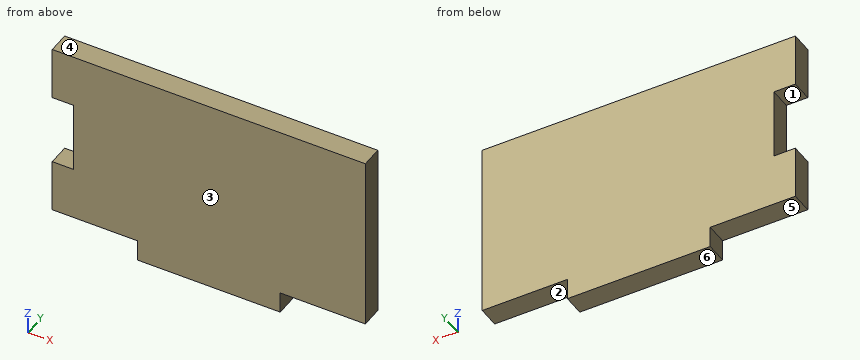
from build123d import *

# Parameters (mm, degrees)
SKETCH1_W           = 23.83759514
SKETCH1_H           = 6
SKETCH1_W_2         = 40
SKETCH1_W_3         = 23.837595139
BOSS_EXTRUDE1_DEPTH = 50
SKETCH1_3_W         = 40
SKETCH1_3_H         = 6
BOSS_EXTRUDE2_DEPTH = 6
SKETCH2_W           = 6
SKETCH2_H           = 20
CUT_EXTRUDE1_DEPTH  = 6


with BuildPart() as part:
    # Sketch1 → Boss-Extrude1 (new body)
    with BuildSketch(Plane.XY):
        with Locations((-42.937060586, -38.008278224)):
            Rectangle(SKETCH1_W, SKETCH1_H)
        with Locations((-11.018263016, -38.008278224)):
            Rectangle(SKETCH1_W_2, SKETCH1_H)
        with Locations((20.900534554, -38.008278224)):
            Rectangle(SKETCH1_W_3, SKETCH1_H)
    extrude(amount=BOSS_EXTRUDE1_DEPTH)

    # Sketch1_3 → Boss-Extrude2 (add)
    with BuildSketch(Plane.XY):
        with Locations((-11.018263016, -38.008278224)):
            Rectangle(SKETCH1_3_W, SKETCH1_3_H)
    extrude(amount=-BOSS_EXTRUDE2_DEPTH)

    # Sketch2 → Cut-Extrude1 (cut)
    with BuildSketch(Plane(origin=(0, -35.008278224, 0), x_dir=(1, 0, 0), z_dir=(0, 1, 0))):
        with Locations((-51.855858156, -25)):
            Rectangle(SKETCH2_W, SKETCH2_H)
    extrude(amount=-CUT_EXTRUDE1_DEPTH, mode=Mode.SUBTRACT)


solid = part.part
Can you work these out from the model? Positions are in its coordinate system, mm. Face numbers are marked on the shaded views. A direction names the side the tool comes from. Round coordinates to 2 decimals unless told otherwise and drop trailing zeros. Order: outer loops, then holes, each group sorted by start corner. A loop starts at its lowest first (then second) coordinate and runs counter-clockwise, first axis right, second up. Notation, with made-up numbers: (35, -37) -> (77, -37) arc R11 cw to (77, -19) -> close; hole circle Ø8 at (66.25, -7.75). An arc over 180 degrees is marked (long way). Write each question's results on one line, items separated by ' | '. Start each with the question number.
Item 1: Will this pin go through, and if not, where does the flat tip stop? pin 1 (3 mm diameter, centred on x = 24, y = -38, fed in from -Z).
Item 2: Please list where these lines run through material, in increasing order: L1, parallel to Z at x = 11, y = -40.2; L2, parallel to X at y = -36.9, z = 28.5; L3, parallel to X at y = -36.8, z = -1.
Item 3: Which directions (+Z, -Z, +X, -X, +Y, -Y) give clear straight access to the entire face, cutting with the end or side of a thin tool? Please do the marked faces 5 and 6.
Item 4: If we section it at C-C, the plane x = -48: Write out the boundary of the cut face in (y, z), then the cut area to 3 significant figures.
Item 5: If we section it at B-B, the plane z = 18.5: Write out the boundary of the cut face in (x, y), then the cut area to 3 significant figures.
Item 6: Thinking about a two-plate mould opening in Z: for the marked faces 1, 2, 3 and 4, which applies, +Z half, -Z half, draft (parallel to the pull), parting line (faces both ways), or undercut?
Item 7: If we section it at A-A, the plane y = -37.45: Write out the boundary of the cut face in (x, z).
Results:
1) pin 1: stops at z = 0
2) L1: z = 0 to 50 | L2: x = -48.86 to 32.82 | L3: x = -31.02 to 8.98
3) face 5: -Z, -X, +Y, -Y | face 6: -Z, +X, -X, +Y, -Y
4) outline: (-41.01, 0) -> (-35.01, 0) -> (-35.01, 50) -> (-41.01, 50) -> close | area: 300 mm2
5) outline: (-48.86, -41.01) -> (32.82, -41.01) -> (32.82, -35.01) -> (-48.86, -35.01) -> close | area: 490 mm2
6) face 1: undercut | face 2: -Z half | face 3: draft | face 4: +Z half
7) outline: (-54.86, 0) -> (-31.02, 0) -> (-31.02, -6) -> (8.98, -6) -> (8.98, 0) -> (32.82, 0) -> (32.82, 50) -> (-54.86, 50) -> (-54.86, 35) -> (-48.86, 35) -> (-48.86, 15) -> (-54.86, 15) -> close
